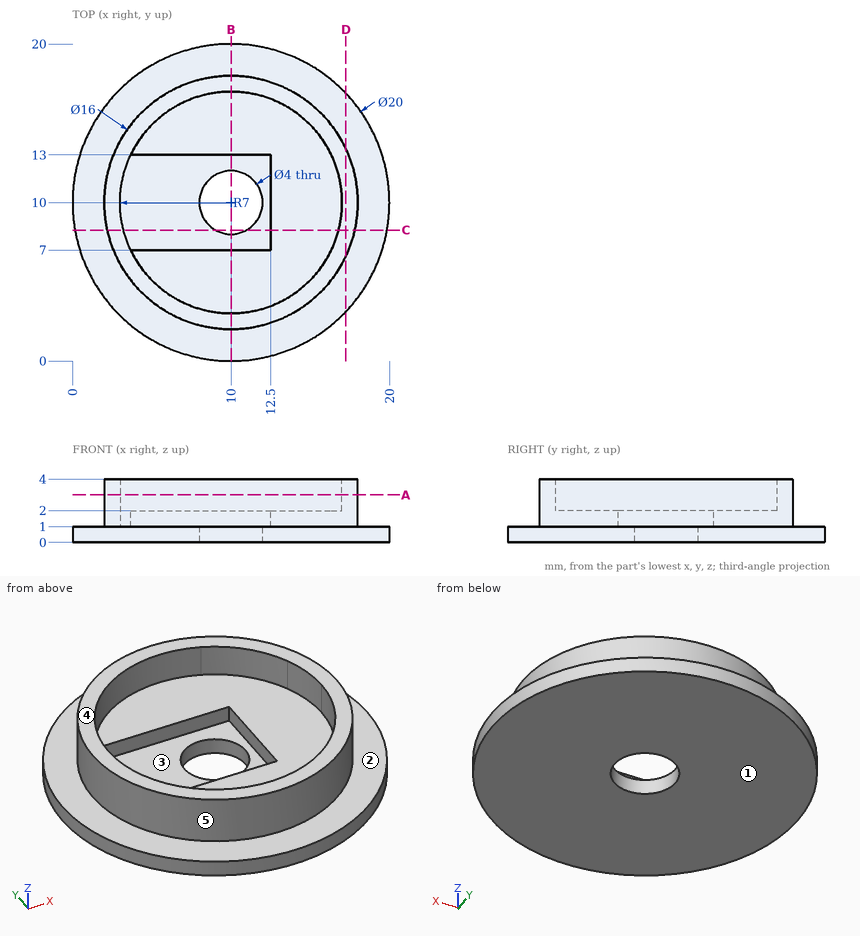
Design review of the part shown in the three views and the two pictorial views. Dimensions are in mm from the part's minimum x, y and z. A direction names the side the tool comes from. Coordinates: 2 decimals unless noted, no trailing zeros. Write each loop counter-clockwise with the first axis right and the second up, starting at its lowest first coordinate (ties: lowest second). Pieces come first, ordered by that corner, then holes. Notation, with made-up numbers: (45.5, -11) -> (91.5, -11) arc R13 cw to (91.5, 11) -> close; hole circle Ø9 at (74, 15). An arc over 180 degrees is marked (long way). Answer in a Markdown table with one row per item.
1. For the marked faces 1 and 2, list the 3-axis set-ups (+Z, -Z, +X, -X, +Y, -Y) from which the entire face can be reached by the end or side of a thin tool; tool diameter is ignored.
Answers below:
| item | result |
|---|---|
| face 1 | -Z, +X, -X, +Y, -Y |
| face 2 | +Z |
2. Draft analysis for pull direction Y (two halves, no side actions). For the marked faces 3, 4 and 5, state which applies: +Y half, -Y half, draft (parallel to the pull), parting line (faces both ways), or undercut.
Answers below:
| item | result |
|---|---|
| face 3 | undercut |
| face 4 | draft |
| face 5 | parting line |
3. We need section C-C, the plane y = 8.25. State the section outline as (x, z) points, and give its area (3 significant figures).
Answers below:
| item | result |
|---|---|
| outline | (0.15, 0) -> (9.03, 0) -> (9.03, 1) -> (3.22, 1) -> (3.22, 4) -> (2.19, 4) -> (2.19, 1) -> (0.15, 1) -> close; (10.97, 0) -> (19.85, 0) -> (19.85, 1) -> (17.81, 1) -> (17.81, 4) -> (16.78, 4) -> (16.78, 2) -> (12.5, 2) -> (12.5, 1) -> (10.97, 1) -> close |
| area | 28.2 mm^2 |
4. Wall thickness on probe 1 along Y at (x, z) = (10, 0.25); probe 2 along Z at (x, y) = (9, 8); probe 3 along Y at (x, z) = (8.75, 3.65): over which ranges is each line inside the solid? List them lowest first. Write a range as [from, to].
Answers below:
| item | result |
|---|---|
| probe 1 | y = [0, 8], [12, 20] |
| probe 2 | z = [0, 1] |
| probe 3 | y = [2.1, 3.11], [16.89, 17.9] |
5. We need section B-B, the plane x = 10. State the section outline as (y, z) points, and give its area (3 significant figures).
Answers below:
| item | result |
|---|---|
| outline | (0, 0) -> (8, 0) -> (8, 1) -> (7, 1) -> (7, 2) -> (3, 2) -> (3, 4) -> (2, 4) -> (2, 1) -> (0, 1) -> close; (12, 0) -> (20, 0) -> (20, 1) -> (18, 1) -> (18, 4) -> (17, 4) -> (17, 2) -> (13, 2) -> (13, 1) -> (12, 1) -> close |
| area | 30.0 mm^2 |
6. We need section D-D, the plane x = 17.25. State the section outline as (y, z) points.
Answers below:
| item | result |
|---|---|
| outline | (3.11, 0) -> (16.89, 0) -> (16.89, 1) -> (13.38, 1) -> (13.38, 4) -> (6.62, 4) -> (6.62, 1) -> (3.11, 1) -> close |
7. We need section A-A, the plane z = 3. State the section outline as (x, y) points, and give its area (3 significant figures).
Answers below:
| item | result |
|---|---|
| outline | circle Ø16 at (10, 10); hole circle Ø14 at (10, 10) |
| area | 47.1 mm^2 |
8. Clearance check with flat-ended pins moving along their axes: pin 1 Ø3 at (x, y) = (2.5, 3.5) entering from -Z; pin 2 Ø0.8 at (x, z) = (9.5, 1.5) entering from -Y; pin 3 Ø3 at (x, y) = (6.5, 9) entering from +Z; pin 4 Ø0.5 at (x, z) = (6.5, 1.5) entering from +Y. State where each tip first meets the part, or that it passes through.
Answers below:
| item | result |
|---|---|
| pin 1 | stops at z = 0 |
| pin 2 | stops at y = 2 |
| pin 3 | stops at z = 1 |
| pin 4 | stops at y = 17.31 |
